```python
from build123d import *

# Parameters (mm, degrees)
EXTRUDE_1_DEPTH          = 5
EXTRUDE_1_DEPTH_BACK     = 7.5
SKETCH_1_W               = 4.5
SKETCH_1_H               = 7
SKETCH_2_W               = 4.5
SKETCH_2_H               = 7
EXTRUDE_2_DEPTH          = 4
FILLET_1_R               = 3
SKETCH_3_W               = 7
SKETCH_3_H               = 4
EXTRUDE_3_DEPTH          = 100
FILLET_2_R               = 5
FILLET_3_R               = 3
CUT_EXTRUDE_1_DEPTH      = 122.436842092
CUT_EXTRUDE_1_DEPTH_BACK = 122.436842092
SKETCH_6_R               = 1.5


with BuildPart() as part:
    # Эскиз1 → Бобышка-Вытянуть1 (new, two sides: drawn at the far end of the back side and taken through both)
    with BuildSketch(Plane(origin=(0, 36.697201552, 0), x_dir=(1, 0, 0), z_dir=(0, 1, 0)).offset(-EXTRUDE_1_DEPTH_BACK)):
        with Locations((-11.75, 0)):
            Rectangle(SKETCH_1_W, SKETCH_1_H)
    extrude(amount=EXTRUDE_1_DEPTH + EXTRUDE_1_DEPTH_BACK)

    # Эскиз2 → Бобышка-Вытянуть2 (add)
    with BuildSketch(Plane.XZ.offset(-29.197201552)):
        with Locations((-11.75, 0)):
            Rectangle(SKETCH_2_W, SKETCH_2_H)
    extrude(amount=-EXTRUDE_2_DEPTH)

    # Скругление1
    fillet_1_edges = [part.edges().sort_by_distance(p)[0] for p in [
        (-9.5, 29.197201552, 0),
    ]]
    fillet(fillet_1_edges, radius=FILLET_1_R)

    # Эскиз3 → Бобышка-Вытянуть3 (add)
    with BuildSketch(Plane.ZY.offset(14)):
        with Locations((0, 31.197201552)):
            Rectangle(SKETCH_3_W, SKETCH_3_H)
    extrude(amount=EXTRUDE_3_DEPTH)

    # Скругление2
    # the kernel refuses this fillet: 5 mm, written as the material it takes off along each edge
    with BuildSketch(Plane(origin=(-9.5, 41.697201552, 15.937342964), x_dir=(-1, 0, 0), z_dir=(0, 0, -1))) as fillet_2_piece_1:
        with BuildLine():
            CenterArc((5, -4.974937186), FILLET_2_R, 95.739170477, 84.260829523)
            Line((0, -4.974937186), (-0.1, -4.974937186))
            Line((-0.1, -4.974937186), (-0.1, 0))
            Line((-0.1, 0), (0, 0.1))
            ThreePointArc((0, 0.1), (2.25, 0.1), (4.49, 0.099498744))
            Line((4.49, 0.099498744), (4.5, 0))
        make_face()
    extrude(amount=31.874685928, mode=Mode.SUBTRACT)

    # Скругление3
    fillet_3_edges = [part.edges().sort_by_distance(p)[0] for p in [
        (-14, 33.197201552, 0),
    ]]
    fillet(fillet_3_edges, radius=FILLET_3_R)

    # Эскиз6 → Вырез-Вытянуть1 (cut, two sides: drawn at the far end of the back side and taken through both)
    with BuildSketch(Plane.XY.offset(-CUT_EXTRUDE_1_DEPTH_BACK)):
        with Locations((-12.5, 32.197201552)):
            Circle(SKETCH_6_R)
    extrude(amount=CUT_EXTRUDE_1_DEPTH + CUT_EXTRUDE_1_DEPTH_BACK, mode=Mode.SUBTRACT)


solid = part.part
```
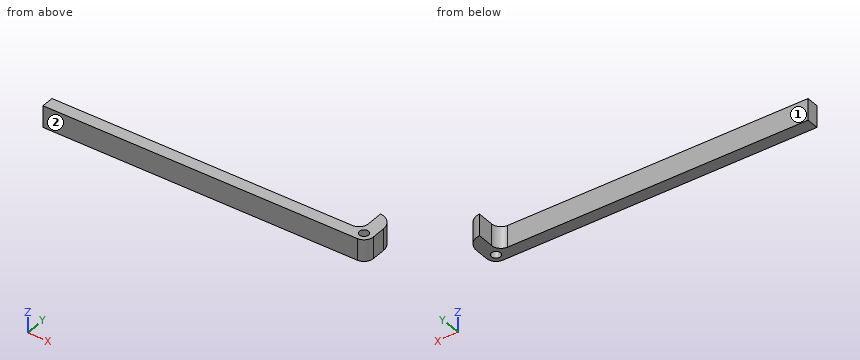
Could you check a few things on this model? Use its own coordinates, in mm. Face numbers are marked on the shaded views. A direction names the side the tool comes from. Give positions to 0.01 mm unless a question says otherwise; leave off trailing zeros. Order: outer loops, then holes, each group sorted by start corner. A loop starts at its lowest first (then second) coordinate and runs counter-clockwise, first axis right, second up.
Q1. I'm going to push flat-ended pins straight in: P1, Ø1.7, axis at y = 39, z = 0.5, coming from the -X side; P2, Ø3.5, axis at x = -56.5, z = 1, coming from the +Y side; P3, Ø1, axis at y = 31.5, z = 1.5, coming from the +X side; P4, Ø2.5, axis at x = -12.5, y = 32.2, coming from the +Z side. Where does each tip first touch, or does it pass through?
Q2. Suppose I cut it at B-B, the plane x = -20.5. Write out the boundary of the cut face in (y, z).
Q3. For the marked faces 1 and 2, which set-ups out of +Z, -Z, +X, -X, +Y, -Y let a thin tool reach every point of the face, with its end or its side?
Q4. Suppose I cut it at C-C, the plane y = 38.75. Write out the boundary of the cut face in (x, z).
Q5. Suppose I cut it at A-A, the plane z = 0.5. Write out the boundary of the cut face in (x, y).
Q6. If I drill on line 1 along X through (y, z) = (32, -3); line 2 along Y through (x, z) = (-66, -0.5); line 3 along X through (y, z) = (31.25, 2.5), over which ranges is the centre line in solid material (lowest first)?
Solution:
1. P1: stops at x = -14
1. P2: stops at y = 33.2
1. P3: stops at x = -9.51
1. P4: passes through
2. outline: (29.2, -3.5) - (33.2, -3.5) - (33.2, 3.5) - (29.2, 3.5) - close
3. face 1: +Z, -Z, -X, +Y
3. face 2: +Z, -Z, +X, -X, -Y
4. outline: (-14, -3.5) - (-9.93, -3.5) - (-9.93, 3.5) - (-14, 3.5) - close
5. outline: (-114, 29.2) - (-12.5, 29.2) arc R3 ccw to (-9.5, 32.2) - (-9.5, 36.72) arc R5 ccw to (-14, 41.7) - (-14, 36.2) arc R3 cw to (-17, 33.2) - (-114, 33.2) - close; hole circle Ø3 at (-12.5, 32.2)
6. line 1: x = -114 to -13.99, -11.01 to -9.51
6. line 2: y = 29.2 to 33.2
6. line 3: x = -114 to -13.66, -11.34 to -9.65
